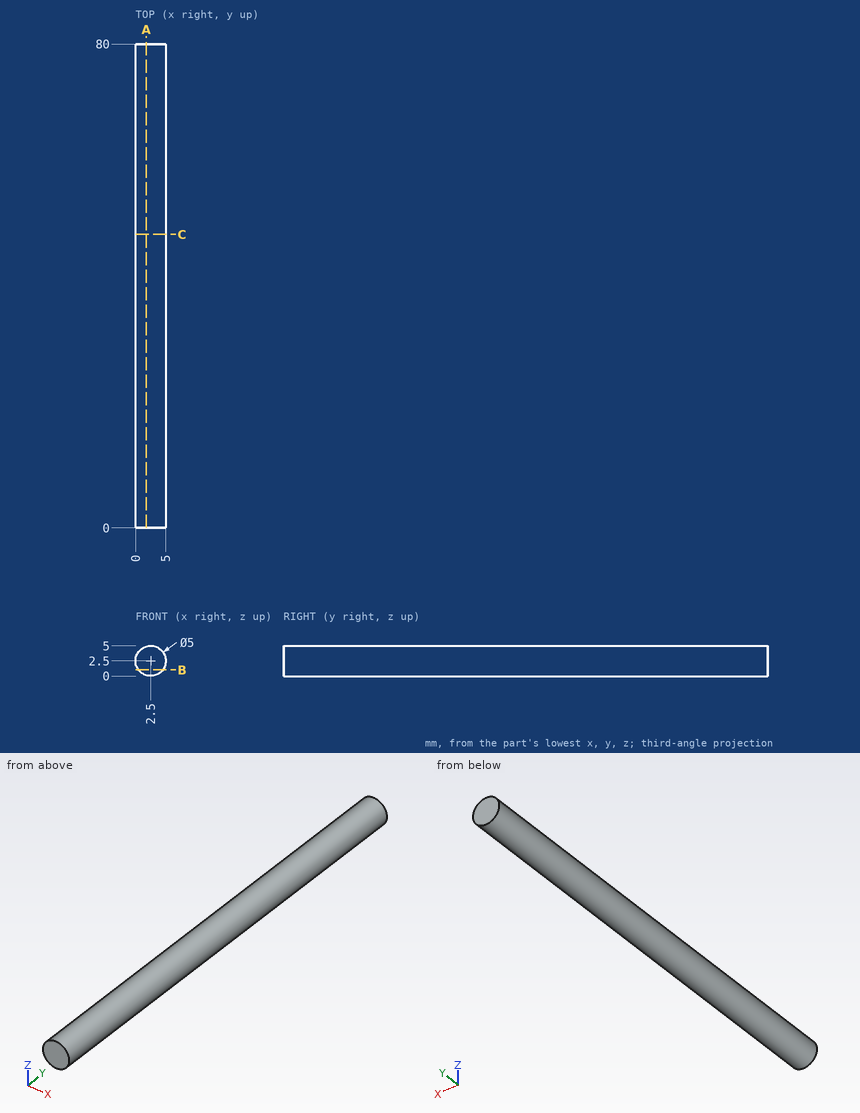
Geometry check sheet. Reference: drawing and pictorial views, mm from the part's lowest x, y, z. Give positions to 0.01 mm unless a question says otherwise; leave off trailing zeros. Loops run counter-clockwise (first coordinate to the right, second up) from the corner with the lowest first, then second, coordinate; pieces in that order, holes last. Notation, with made-up numbers: (2.25, -20) - (52.25, -20) arc R16 cw to (52.25, 5) - close; hole circle Ø5 at (73, 66.5). An arc over 180 degrees is marked (long way). One line per question, with ' | ' between items. Start each with the question number.
1. Cross-section at C-C, the plane y = 48.5. Enter the section's corners in (x, z), plus the area to 3 significant figures.
2. Cross-section at A-A, the plane x = 1.8. Enter the section's corners in (y, z), plus the area to 3 significant figures.
3. Material ranges on line 1 along Z through (x, y) = (2.7, 5.5); line 2 along Z through (x, y) = (1.65, 67); line 3 along X through (y, z) = (16.5, 1.5), recorded low to high. Write a range as [from, to].
4. Gauge pin test, flat end, axial feed: pin 1 Ø2 at (x, y) = (4, 28) entering from -Z. Record the tip position at first contact, or that the pin passes through.
5. Cross-section at B-B, the plane z = 1. Enter the section's corners in (x, y).
Check result:
1) outline: circle Ø5 at (2.5, 2.5) | area: 19.6 mm2
2) outline: (0, 0.1) - (80, 0.1) - (80, 4.9) - (0, 4.9) - close | area: 384 mm2
3) line 1: z = [0.01, 4.99] | line 2: z = [0.15, 4.85] | line 3: x = [0.21, 4.79]
4) pin 1: stops at z = 0.05
5) outline: (0.5, 0) - (4.5, 0) - (4.5, 80) - (0.5, 80) - close
